```python
from build123d import *
from build123d.topology import SkipClean

# Parameters (mm, degrees)
EXTRUDE_START            = 1.5
EXTRUDE_4_DEPTH          = 1.5
EXTRUDE_START_2          = 10.5
EXTRUDE_5_DEPTH          = 10.5
PATTERN_CIRCULAR_2_COUNT = 2
CUT_EXTRUDE_3_DEPTH      = 53.692504211


with BuildPart() as part:
    # Эскиз1 → Повернуть1 (revolve)
    with BuildSketch(Plane.XY, mode=Mode.PRIVATE) as revolve_1_sk:
        Polygon((0, 22.5), (0, 7), (30, 7), (30, 13), (4, 13), (4, 22.5), align=None)
    revolve(revolve_1_sk.sketch.rotate(Axis((0, 0, 0), (1, 0, 0)), 90), axis=Axis((0, 0, 0), (1, 0, 0)))

    # Эскиз7 → Бобышка-Вытянуть4 (add)
    with BuildSketch(Plane.ZY.offset(EXTRUDE_START)):
        with BuildLine():
            Line((0, 22.5), (0, 14.142135624))
            Line((0, 14.142135624), (14.142135624, 0))
            Line((14.142135624, 0), (22.5, 0))
            ThreePointArc((22.5, 0), (15.909902577, 15.909902577), (0, 22.5))
        make_face()
    extrude_4 = extrude(amount=-EXTRUDE_4_DEPTH)

    # Эскиз9 → Бобышка-Вытянуть5 (add)
    with BuildSketch(Plane.ZY.offset(1.5).offset(EXTRUDE_START_2)):
        with BuildLine():
            Line((5, 21.937410968), (5, 9.142135624))
            Line((5, 9.142135624), (9.142135624, 5))
            Line((9.142135624, 5), (21.937410968, 5))
            ThreePointArc((21.937410968, 5), (15.909902577, 15.909902577), (5, 21.937410968))
        make_face()
    extrude_5 = extrude(amount=-EXTRUDE_5_DEPTH)

    # Круговой массив2: Бобышка-Вытянуть4, Бобышка-Вытянуть5 ×2 about axis
    with SkipClean():  # the faces are left unmerged after this step: merging them gives an invalid solid
        pattern_circular_2_axis = Axis((0, 0, 0), (1, 0, 0))
        add([extrude_4.rotate(pattern_circular_2_axis, i * 360 / PATTERN_CIRCULAR_2_COUNT) for i in range(1, PATTERN_CIRCULAR_2_COUNT)])
        add([extrude_5.rotate(pattern_circular_2_axis, i * 360 / PATTERN_CIRCULAR_2_COUNT) for i in range(1, PATTERN_CIRCULAR_2_COUNT)])

    # Эскиз10 → Вырез-Вытянуть3 (cut, through all)
    with SkipClean():  # the faces are left unmerged after this step: merging them gives an invalid solid
        with BuildSketch(Plane(origin=(30, 0, 0), x_dir=(0, 0, -1), z_dir=(1, 0, 0))):
            Polygon((1.767766953, -1.767766953), (-1.767766953, 1.767766953), (-8.343860018, -4.808326112), (-4.808326112, -8.343860018), align=None)
        extrude(amount=-CUT_EXTRUDE_3_DEPTH, mode=Mode.SUBTRACT)


solid = part.part
```
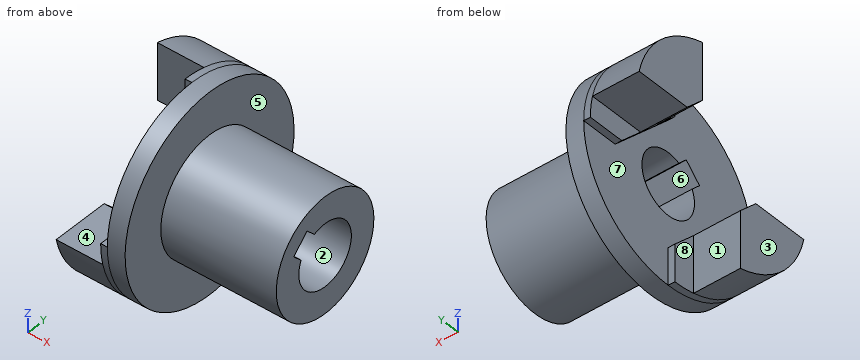
Here's how the part is built. I have some questions about the finished solid (model axes, mm). Face numbers are marked on the shaded views. A direction names the side the tool comes from. Round coordinates to 2 decimals unless told otherwise and drop trailing zeros. Write each loop counter-clockwise with the first axis right and the second up, starting at its lowest first coordinate (ties: lowest second). Pieces come first, ordered by that corner, then holes.
Q1. If we section it at B-B on y = 3: Write out the boundary of the cut face in (x, z).
Q2. Which directions (+Z, -Z, +X, -X, +Y, -Y) give clear straight access to the entire face, cutting with the end or side of a thin tool? Please do the marked faces 4, 5, 6, 7 and 8.
Q3. If we mould it in two halves opening along Y, with no side actions, what happens to the marked faces 1, 2 and 3? For each: +Y half, -Y half, draft (parallel to the pull), parting line (faces both ways), or undercut.
Q4. If we section it at D-D on z = 17: Write out the boundary of the cut face in (x, y).
Q5. Please list where these lines run through material, in increasing order: probe 1 along Y at (x, z) = (23, 0); probe 2 along X at (y, z) = (-20, -0.5); probe 3 along X at (y, z) = (13, 15).
Q6. If we section it at C-C on y = 19: Write out the boundary of the cut face in (x, z), plus the area to 3 significant figures.
Q7. If we section it at A-A on x = 22: Write out the boundary of the cut face in (y, z), plus the area to 3 significant figures.
Q8. Will these pins go through, and if not, where does the flat tip stop? P1, Ø3, axis at x = -7, z = -16, coming from the +Y side; P2, Ø0.8, axis at x = -0.5, z = -17.5, coming from the +Y side; P3, Ø0.8, axis at x = -1, y = -16.5, coming from the +Z side; P4, Ø11, axis at y = 0, z = 0, coming from the +X side.
Answer below:
1. outline: (-1.5, 11.14) - (0, 11.14) - (0, 6.32) - (30, 6.32) - (30, 12.65) - (4, 12.65) - (4, 22.3) - (-1.5, 22.3) - close; (0, -22.3) - (4, -22.3) - (4, -12.65) - (30, -12.65) - (30, -6.32) - (0, -6.32) - close
2. face 4: +Z, -X, +Y, -Y
2. face 5: +X
2. face 6: +X, -X
2. face 7: -X
2. face 8: +Z, -Z, -X, +Y
3. face 1: +Y half
3. face 2: undercut
3. face 3: draft
4. outline: (-12, 5) - (-1.5, 5) - (-1.5, 0) - (0, 0) - (0, -14.74) - (4, -14.74) - (4, 14.74) - (-12, 14.74) - close
5. probe 1: y = -13 to -7, 7 to 13
5. probe 2: x = -1.5 to 4
5. probe 3: x = -12 to 4
6. outline: (-12, 5) - (-1.5, 5) - (-1.5, 0) - (0, 0) - (0, -12.05) - (4, -12.05) - (4, 12.05) - (-12, 12.05) - close
6. area: 189 mm2
7. outline: circle Ø26 at (0, 0); hole (-8.34, 4.81) - (-6.39, 2.86) arc R7 ccw (long way) to (-2.86, 6.39) - (-4.81, 8.34) - close
7. area: 365 mm2
8. P1: stops at y = -5
8. P2: stops at y = 0
8. P3: stops at z = 0
8. P4: passes through
